Drawing for the job (mm, zero at the part's lowest x, y, z). A direction names the side the tool comes from. Give positions to 0.01 mm unless a question says otherwise; leave off trailing zeros. Order: outer loops, then holes, each group sorted by start corner. A loop starts at its lowest first (then second) coordinate and runs counter-clockwise, first axis right, second up. Notation, with made-up numbers: (-1, 56) - (17, 56) arc R16 ccw to (17, 76) - close; hole circle Ø5 at (36, 13). An arc over 180 degrees is marked (long way). Use CSV: the item, a comma, the result in double quotes. Start each with the question number.
(1) Band-saw the part on B-B, the plane y = 13. Give the cut face in (x, z).
(2) Drop flat-ended pins along their axis: pin 1 Ø9 at (x, y) = (132.5, 25) entering from +Z; pin 2 Ø4 at (y, z) = (16, 10.5) entering from -X; pin 3 Ø8 at (x, z) = (30, 16) entering from -Y. Give the stop position or say it passes through.
(3) Band-saw the part on A-A, the plane z = 7. Give the cut face in (x, y).
(4) Probe L1, parallel to Y at x = 163.5, z = 10.5; L2, parallel to Z at x = 39, y = 31; L3, parallel to X at y = 30, z = 9.75. List the from-to ranges inside material, lowest first.
(5) Tool access for the marked faces 1 and 2: list every direction of +Z, -Z, +X, -X, +Y, -Y with a clear straight run to the whole face (end or side of a thin tool).
(6) Band-saw the part on C-C, the plane x = 34. Give the cut face in (y, z), then the cut area to 3 significant figures.
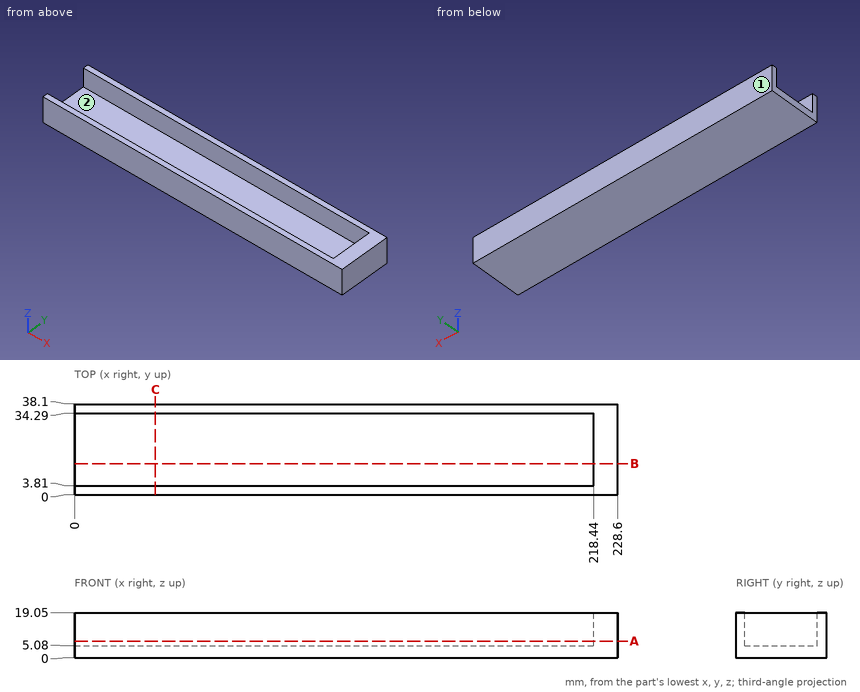
Answer block:
1,outline,"(0, 0) - (228.6, 0) - (228.6, 19.05) - (218.44, 19.05) - (218.44, 5.08) - (0, 5.08) - close"
2,pin 1,"stops at z = 5.08"
2,pin 2,"stops at x = 218.44"
2,pin 3,"stops at y = 0"
3,outline,"(0, 0) - (228.6, 0) - (228.6, 38.1) - (0, 38.1) - (0, 34.29) - (218.44, 34.29) - (218.44, 3.81) - (0, 3.81) - close"
4,L1,"y = 0 to 3.81, 34.29 to 38.1"
4,L2,"z = 0 to 5.08"
4,L3,"x = 218.44 to 228.6"
5,face 1,"+Z, -Z, +X, -X, +Y"
5,face 2,"+Z, -X"
6,outline,"(0, 0) - (38.1, 0) - (38.1, 19.05) - (34.29, 19.05) - (34.29, 5.08) - (3.81, 5.08) - (3.81, 19.05) - (0, 19.05) - close"
6,area,"300 mm2"
